```python
from build123d import *

# Parameters (mm, degrees)
F0_W     = 50
F0_H     = 50
F1_DEPTH = 40
F4_DEPTH = 25
F6_DEPTH = 40.0010001
F7_DEPTH = 40.0010001


with BuildPart() as f1:
    # F0 (on Front) → F1 (new body, symmetric)
    with BuildSketch(Plane.XZ):
        Rectangle(F0_W, F0_H)
    extrude(amount=F1_DEPTH, both=True)

    # F3 (on offset) → F4 (cut)
    with BuildSketch(Plane.YZ.offset(25)):
        with BuildLine():
            Line((20, -25.4437979311), (0, -25.4437979311))
            Line((0, -25.4437979311), (-20, -25.4437979311))
            add(Edge.make_bspline(
                [(20, -25.4437979311), (12.4066961802, -39.0920548923), (-12.4066961802, -39.0920548923), (-20, -25.4437979311)],
                knots=[0.6990551923, 0.6990551923, 0.6990551923, 0.6990551923, 1, 1, 1, 1], degree=3))
        make_face()
        with BuildLine():
            Line((-20, -25.4437979311), (0, -25.4437979311))
            Line((0, -25.4437979311), (20, -25.4437979311))
            add(Edge.make_bspline(
                [(-20, -25.4437979311), (-28.819122854, -9.5922453342), (0, 58.9319309233), (28.819122854, -9.5922453342), (20, -25.4437979311)],
                knots=[0, 0, 0, 0, 0.3495275962, 0.6990551923, 0.6990551923, 0.6990551923, 0.6990551923], degree=3))
        make_face()
    extrude(amount=-F4_DEPTH, mode=Mode.SUBTRACT)

    # F5 (on Front) → F6 (cut, through all)
    with BuildSketch(Plane.XZ):
        Polygon((-6, 20), (-30, 20), (-30, -20), (-6, -20), (-6, 0), align=None)
    extrude(amount=-F6_DEPTH, mode=Mode.SUBTRACT)

    # F5 (on Front) → F7 (cut, through all)
    with BuildSketch(Plane.XZ):
        Polygon((-6, 20), (-30, 20), (-30, -20), (-6, -20), (-6, 0), align=None)
    extrude(amount=F7_DEPTH, mode=Mode.SUBTRACT)


solid = f1.part
```
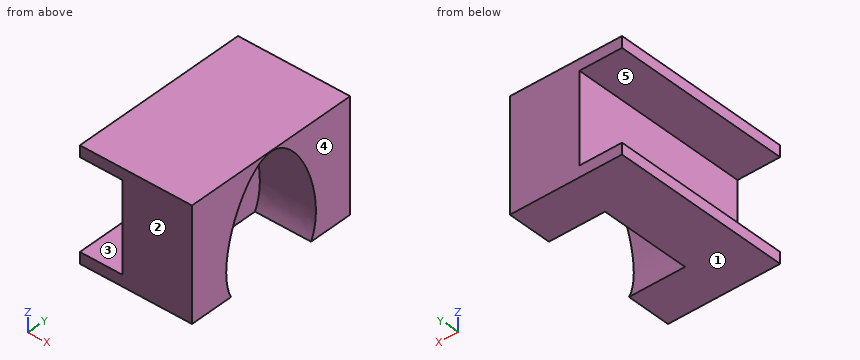
Check sheet for the modelled part. Datum: model origin and axes. Units: mm. Face numbers are marked on the shaded views. A direction names the side the tool comes from. Coordinates: 2 decimals unless noted, no trailing zeros. Loops run counter-clockwise (first coordinate to the right, second up) from the corner with the lowest first, then second, coordinate; pieces in that order, holes last.
1) Sectioned sample at A-A (x = -10.5). Record the boundary of the cut face in (y, z), and give its area (3 significant figures).
2) Release check for a two-part mould opening along Z. For the marked faces 1, 2 and 3 record: released by +Z, released by -Z, zero draft, split by the parting line, or undercut.
3) Sectioned sample at B-B (y = 34). Record the boundary of the cut face in (x, z).
4) Material ranges on probe 1 along Y at (x, z) = (13, -13); probe 2 along Z at (x, y) = (-17.5, 27); probe 3 along X at (y, z) = (14, 10.5), recorded low to high.
5) Gauge pin test, flat ends, axial feed: pin 1 (8 mm diameter, centred on x = 10, y = 4.5, fed in from -Z); pin 2 (2 mm diameter, centred on y = 0.5, z = 5.5, fed in from -X). Record the tip position at first contact, or that the pin passes through.
6) Access from +Z, -Z, +X, -X, +Y, -Y to the whole of each face (thin tool, end or side, straight path). Record for the marked faces 4 and 5.
Check sheet entries:
1. outline: (-40, -25) - (40, -25) - (40, -20) - (-40, -20) - close; (-40, 20) - (40, 20) - (40, 25) - (-40, 25) - close
1. area: 800 mm2
2. face 1: released by -Z
2. face 2: zero draft
2. face 3: undercut
3. outline: (-25, -25) - (25, -25) - (25, 25) - (-25, 25) - (-25, 20) - (-6, 20) - (-6, -20) - (-25, -20) - close
4. probe 1: y = -40 to -22.7, 22.7 to 40
4. probe 2: z = -25 to -20, 20 to 25
4. probe 3: x = -6 to 0
5. pin 1: stops at z = 20.95
5. pin 2: stops at x = -6
6. face 4: +Z, -Z, +X, +Y, -Y
6. face 5: -X, +Y, -Y
